```python
from build123d import *

# Parameters (mm, degrees)
BOSS_EXTRUDE1_DEPTH     = 9
SKETCH4_R               = 3.1
BOSS_EXTRUDE3_DEPTH     = 1.75
BOSS_EXTRUDE3_DRAFT     = 35
SKETCH7_R               = 1.600000259
CUT_EXTRUDE4_DEPTH      = 15
CUT_EXTRUDE5_DEPTH      = 7
MIRROR1_START           = -14
MIRROR1_DEPTH           = 4
MIRROR1_START_2         = -18.75
MIRROR1_2_OUTLINE_R     = 1.600000259
MIRROR1_2_DEPTH         = 4.75
CIRPATTERN1_START       = -14
CIRPATTERN1_DEPTH       = 28
CIRPATTERN1_START_2     = -18.75
CIRPATTERN1_2_OUTLINE_R = 1.600000259
CIRPATTERN1_2_DEPTH     = 37.5
CIRPATTERN1_START_3     = -20.405762011
CIRPATTERN1_3_OUTLINE_R = 1.600000259
CIRPATTERN1_3_DEPTH     = 1.655762011
CIRPATTERN1_4_DEPTH     = 28
CIRPATTERN1_5_OUTLINE_R = 1.600000259
CIRPATTERN1_5_DEPTH     = 37.5
CIRPATTERN1_START_4     = 18.75
CIRPATTERN1_6_OUTLINE_R = 1.600000259
CIRPATTERN1_6_DEPTH     = 1.616403084
SKETCH8_R               = 11.1
CUT_EXTRUDE6_DEPTH      = 55.051282913
CUT_EXTRUDE6_TAPER      = 2
SKETCH9_R               = 1.6
CUT_EXTRUDE8_DEPTH      = 55.051282913
CHAMFER1_SIZE           = 1.036815955
CHAMFER1_SIZE_2         = 1


with BuildPart() as part:
    # Sketch3 → Boss-Extrude1 (new body)
    with BuildSketch(Plane.XY):
        with BuildLine():
            Line((-18.75, -34.5), (-18.75, -25.5))
            ThreePointArc((-18.75, -25.5), (-22.155271914, -12.791352203), (-31.458647797, -3.487976321))
            Line((-31.458647797, -3.487976321), (-39.252876431, 1.012023679))
            ThreePointArc((-39.252876431, 1.012023679), (-39.718802257, 1.619230038), (-39.618901834, 2.378049083))
            Line((-39.618901834, 2.378049083), (-36.243901834, 8.223720558))
            ThreePointArc((-36.243901834, 8.223720558), (-35.636695476, 8.689646385), (-34.877876431, 8.589745962))
            Line((-34.877876431, 8.589745962), (-27.9496732, 4.589745962))
            ThreePointArc((-27.9496732, 4.589745962), (-26.811444633, 4.439895328), (-25.900635095, 5.138784068))
            Line((-25.900635095, 5.138784068), (-17.400635095, 19.861215932))
            ThreePointArc((-17.400635095, 19.861215932), (-17.250784461, 20.9994445), (-17.9496732, 21.910254038))
            Line((-17.9496732, 21.910254038), (-24.877876431, 25.910254038))
            ThreePointArc((-24.877876431, 25.910254038), (-25.343802257, 26.517460397), (-25.243901834, 27.276279442))
            Line((-25.243901834, 27.276279442), (-21.868901834, 33.121950917))
            ThreePointArc((-21.868901834, 33.121950917), (-21.261695476, 33.587876743), (-20.502876431, 33.487976321))
            Line((-20.502876431, 33.487976321), (-12.708647797, 28.987976321))
            ThreePointArc((-12.708647797, 28.987976321), (0, 25.582704407), (12.708647797, 28.987976321))
            Line((12.708647797, 28.987976321), (20.502876431, 33.487976321))
            ThreePointArc((20.502876431, 33.487976321), (21.261695476, 33.587876743), (21.868901834, 33.121950917))
            Line((21.868901834, 33.121950917), (25.243901834, 27.276279442))
            ThreePointArc((25.243901834, 27.276279442), (25.343802257, 26.517460397), (24.877876431, 25.910254038))
            Line((24.877876431, 25.910254038), (17.9496732, 21.910254038))
            ThreePointArc((17.9496732, 21.910254038), (17.250784461, 20.9994445), (17.400635095, 19.861215932))
            Line((17.400635095, 19.861215932), (25.900635095, 5.138784068))
            ThreePointArc((25.900635095, 5.138784068), (26.811444633, 4.439895328), (27.9496732, 4.589745962))
            Line((27.9496732, 4.589745962), (34.877876431, 8.589745962))
            ThreePointArc((34.877876431, 8.589745962), (35.636695476, 8.689646385), (36.243901834, 8.223720558))
            Line((36.243901834, 8.223720558), (39.618901834, 2.378049083))
            ThreePointArc((39.618901834, 2.378049083), (39.718802257, 1.619230038), (39.252876431, 1.012023679))
            Line((39.252876431, 1.012023679), (31.458647797, -3.487976321))
            ThreePointArc((31.458647797, -3.487976321), (22.155271914, -12.791352203), (18.75, -25.5))
            Line((18.75, -25.5), (18.75, -34.5))
            ThreePointArc((18.75, -34.5), (18.457106781, -35.207106781), (17.75, -35.5))
            Line((17.75, -35.5), (11, -35.5))
            ThreePointArc((11, -35.5), (10.292893219, -35.207106781), (10, -34.5))
            Line((10, -34.5), (10, -19))
            ThreePointArc((10, -19), (9.560660172, -17.939339828), (8.5, -17.5))
            Line((8.5, -17.5), (-8.5, -17.5))
            ThreePointArc((-8.5, -17.5), (-9.560660172, -17.939339828), (-10, -19))
            Line((-10, -19), (-10, -34.5))
            ThreePointArc((-10, -34.5), (-10.292893219, -35.207106781), (-11, -35.5))
            Line((-11, -35.5), (-17.75, -35.5))
            ThreePointArc((-17.75, -35.5), (-18.457106781, -35.207106781), (-18.75, -34.5))
        make_face()
    extrude(amount=BOSS_EXTRUDE1_DEPTH)


with BuildPart() as boss_extrude3_tool:
    # Sketch4 → Boss-Extrude3 (with draft: the straight prism first)
    with BuildSketch(Plane(origin=(20.5, 0, 0), x_dir=(0, 0, -1), z_dir=(1, 0, 0))):
        with Locations((-4.5, -30)):
            Circle(SKETCH4_R)
    extrude(amount=-BOSS_EXTRUDE3_DEPTH)
    # Boss-Extrude3: the draft: its side faces are tilted about the plane it starts from
    boss_extrude3_sides = [boss_extrude3_tool.faces().sort_by_distance(p)[0] for p in [
        (19.625, -30, 7.6),
    ]]
    draft(boss_extrude3_sides, Plane(origin=(20.5, 0, 0), x_dir=(0, 0, -1), z_dir=(1, 0, 0)), BOSS_EXTRUDE3_DRAFT)


with BuildPart() as part_1:
    add(part.part)

    # Boss-Extrude3: add boss_extrude3_tool
    add(boss_extrude3_tool.part)

    # Sketch7 → Cut-Extrude4 (cut)
    with BuildSketch(Plane(origin=(20.5, 0, 0), x_dir=(0, 0, -1), z_dir=(1, 0, 0))):
        with Locations((-4.5, -30)):
            Circle(SKETCH7_R)
    extrude(amount=-CUT_EXTRUDE4_DEPTH, mode=Mode.SUBTRACT)

    # Sketch5 → Cut-Extrude5 (cut)
    with BuildSketch(Plane(origin=(14, 0, 0), x_dir=(0, 0, -1), z_dir=(1, 0, 0))):
        Polygon((-7.349999794, -28.354551852), (-7.349999794, -31.645448148), (-4.5, -33.290896297), (-1.650000206, -31.645448148), (-1.650000206, -28.354551852), (-4.5, -26.709103703), align=None)
    extrude(amount=-CUT_EXTRUDE5_DEPTH, mode=Mode.SUBTRACT)

    # Mirror1: read off the stored shape, not the designer's step
    # Mirror1 outline → Mirror1 (cut)
    with BuildSketch(Plane.YZ.offset(MIRROR1_START)):
        Polygon((-26.709103703, 4.5), (-28.354551852, 7.349999794), (-31.645448148, 7.349999794), (-33.290896297, 4.5), (-31.645448148, 1.650000206), (-28.354551852, 1.650000206), align=None)
    extrude(amount=MIRROR1_DEPTH, mode=Mode.SUBTRACT)

    # Mirror1 2 outline → Mirror1 2 (cut)
    with BuildSketch(Plane.YZ.offset(MIRROR1_START_2)):
        with Locations((-30, 4.5)):
            Circle(MIRROR1_2_OUTLINE_R)
    extrude(amount=MIRROR1_2_DEPTH, mode=Mode.SUBTRACT)

    # Mirror1 3 outline → Mirror1 3 (revolve)
    with BuildSketch(Plane(origin=(0, -30, 4.5), x_dir=(0, 1, 0), z_dir=(0, 0, -1))):
        Polygon((1.600000259, -18.75), (1.600000259, -20.5), (3.1, -20.5), (4.325363192, -18.75), align=None)
    revolve(axis=Axis((0, -30, 4.5), (1, 0, 0)))

    # CirPattern1: read off the stored shape, not the designer's step
    # CirPattern1 outline → CirPattern1 (cut)
    with BuildSketch(Plane(origin=(0, 0, 0), x_dir=(0.8660254037844362, 0.5000000000000042, 0), z_dir=(0.5000000000000042, -0.8660254037844363, 0)).offset(CIRPATTERN1_START)):
        Polygon((26.709103703, 4.5), (28.354551852, 1.650000206), (31.645448148, 1.650000206), (33.290896297, 4.5), (31.645448148, 7.349999794), (28.354551852, 7.349999794), align=None)
    extrude(amount=CIRPATTERN1_DEPTH, mode=Mode.SUBTRACT)

    # CirPattern1 2 outline → CirPattern1 2 (cut)
    with BuildSketch(Plane(origin=(0, 0, 0), x_dir=(0.8660254037844362, 0.5000000000000042, 0), z_dir=(0.5000000000000042, -0.8660254037844363, 0)).offset(CIRPATTERN1_START_2)):
        with Locations((30, 4.5)):
            Circle(CIRPATTERN1_2_OUTLINE_R)
    extrude(amount=CIRPATTERN1_2_DEPTH, mode=Mode.SUBTRACT)

    # CirPattern1 3 outline → CirPattern1 3 (add)
    with BuildSketch(Plane(origin=(0, 0, 0), x_dir=(0.8660254037844362, 0.5000000000000042, 0), z_dir=(0.5000000000000042, -0.8660254037844363, 0)).offset(CIRPATTERN1_START_3)):
        Polygon((26.709103703, 4.5), (28.354551852, 1.650000206), (31.645448148, 1.650000206), (33.290896297, 4.5), (31.645448148, 7.349999794), (28.354551852, 7.349999794), align=None)
        with Locations((30, 4.5)):
            Circle(CIRPATTERN1_3_OUTLINE_R, mode=Mode.SUBTRACT)
    extrude(amount=CIRPATTERN1_3_DEPTH)

    # CirPattern1 4 outline → CirPattern1 4 (cut)
    with BuildSketch(Plane(origin=(0, 0, 0), x_dir=(0.8660254037844431, -0.4999999999999921, 0), z_dir=(0.4999999999999921, 0.8660254037844433, 0)).offset(CIRPATTERN1_START)):
        Polygon((-26.709103703, -4.5), (-28.354551852, -1.650000206), (-31.645448148, -1.650000206), (-33.290896297, -4.5), (-31.645448148, -7.349999794), (-28.354551852, -7.349999794), align=None)
    extrude(amount=CIRPATTERN1_4_DEPTH, mode=Mode.SUBTRACT)

    # CirPattern1 5 outline → CirPattern1 5 (cut)
    with BuildSketch(Plane(origin=(0, 0, 0), x_dir=(0.8660254037844431, -0.4999999999999921, 0), z_dir=(0.4999999999999921, 0.8660254037844433, 0)).offset(CIRPATTERN1_START_2)):
        with Locations((-30, -4.5)):
            Circle(CIRPATTERN1_5_OUTLINE_R)
    extrude(amount=CIRPATTERN1_5_DEPTH, mode=Mode.SUBTRACT)

    # CirPattern1 6 outline → CirPattern1 6 (add)
    with BuildSketch(Plane(origin=(0, 0, 0), x_dir=(0.8660254037844431, -0.4999999999999921, 0), z_dir=(0.4999999999999921, 0.8660254037844433, 0)).offset(CIRPATTERN1_START_4)):
        Polygon((-26.709103703, -4.5), (-28.354551852, -1.650000206), (-31.645448148, -1.650000206), (-33.290896297, -4.5), (-31.645448148, -7.349999794), (-28.354551852, -7.349999794), align=None)
        with Locations((-30, -4.5)):
            Circle(CIRPATTERN1_6_OUTLINE_R, mode=Mode.SUBTRACT)
    extrude(amount=CIRPATTERN1_6_DEPTH)

    # CirPattern1 7 outline → CirPattern1 7 (revolve)
    with BuildSketch(Plane(origin=(-25.980762114, 15, 4.5), x_dir=(0.8660254037844431, -0.4999999999999921, 0), z_dir=(0, 0, 1))):
        Polygon((3.1, 20.5), (1.600000259, 20.5), (1.600000259, 18.75), (4.325363192, 18.75), align=None)
        Polygon((1.600000259, -18.75), (1.600000259, -20.5), (3.1, -20.5), (4.325363192, -18.75), align=None)
    revolve(axis=Axis((-25.980762114, 15, 4.5), (0.4999999999999921, 0.8660254037844431, 0)))

    # CirPattern1 8 outline → CirPattern1 8 (revolve)
    with BuildSketch(Plane(origin=(25.980762114, 15, 4.5), x_dir=(0.8660254037844362, 0.5000000000000042, 0), z_dir=(0, 0, -1))):
        Polygon((3.1, 20.5), (1.600000259, 20.5), (1.600000259, 18.75), (4.325363192, 18.75), align=None)
        Polygon((1.600000259, -18.75), (1.600000259, -20.5), (3.1, -20.5), (4.325363192, -18.75), align=None)
    revolve(axis=Axis((25.980762114, 15, 4.5), (0.5000000000000042, -0.8660254037844362, 0)))

    # CirPattern1 9 outline → CirPattern1 9 (revolve, cut)
    with BuildSketch(Plane(origin=(-25.980762114, 15, 4.5), x_dir=(0.8660254037844431, -0.4999999999999921, 0), z_dir=(0, 0, 1))):
        Polygon((3.290896297, 20.366403084), (3.193545568, 20.366403084), (3.290896297, 20.227371834), align=None)
    revolve(axis=Axis((-25.980762114, 15, 4.5), (0.4999999999999921, 0.8660254037844431, 0)), mode=Mode.SUBTRACT)

    # CirPattern1 10 outline → CirPattern1 10 (revolve, cut)
    with BuildSketch(Plane(origin=(25.980762114, 15, 4.5), x_dir=(0.8660254037844362, 0.5000000000000042, 0), z_dir=(0, 0, -1))):
        Polygon((3.290896297, -20.227371834), (3.16598615, -20.405762011), (3.290896297, -20.405762011), align=None)
    revolve(axis=Axis((25.980762114, 15, 4.5), (0.5000000000000042, -0.8660254037844362, 0)), mode=Mode.SUBTRACT)

    # Sketch8 → Cut-Extrude6 (cut, through all)
    with BuildSketch(Plane.XY):
        Circle(SKETCH8_R)
    extrude(amount=CUT_EXTRUDE6_DEPTH, taper=CUT_EXTRUDE6_TAPER, mode=Mode.SUBTRACT)

    # Sketch9 → Cut-Extrude8 (cut, through all)
    with BuildSketch(Plane.XY):
        with Locations((13.1, -7.1)):
            Circle(SKETCH9_R)
        with Locations((13.1, 7.1)):
            Circle(SKETCH9_R)
        with Locations((-13.1, 7.1)):
            Circle(SKETCH9_R)
        with Locations((-13.1, -7.1)):
            Circle(SKETCH9_R)
    extrude(amount=CUT_EXTRUDE8_DEPTH, mode=Mode.SUBTRACT)

    # Chamfer1
    # the kernel refuses this chamfer: 1.036815955, 1 mm, written as the material it takes off along each edge
    with BuildSketch(Plane(origin=(0, 0, 0), x_dir=(1, 0, 0), z_dir=(0, 1, 0))) as chamfer1_piece_1:
        Polygon((11.1 + CHAMFER1_SIZE, 0), (11.1 - CHAMFER1_SIZE_2 * 0.0348994967025, -CHAMFER1_SIZE_2 * 0.999390827019), (11.1, 0), align=None)
    revolve(axis=Axis((0, 0, 0), (0, 0, -1)), mode=Mode.SUBTRACT)


solid = part_1.part
```
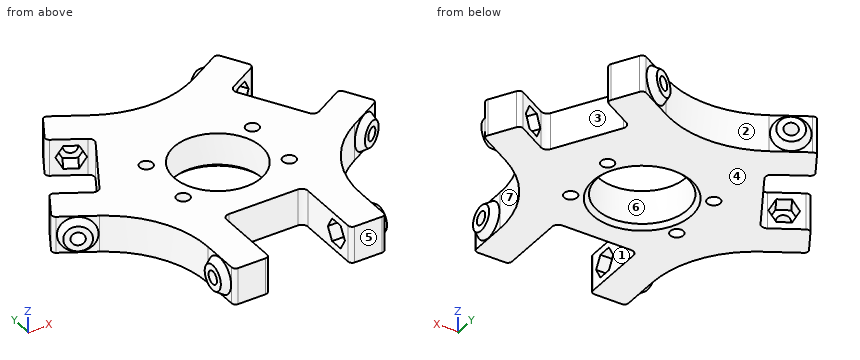
The listing builds one solid part. Answer for the finished solid, in the listing's coordinates (mm). Face numbers are marked on the shaded views. A direction names the side the tool comes from. Coordinates: 2 decimals unless noted, no trailing zeros. Write each loop counter-clockwise with the first axis right and the second up, starting at its lowest first coordinate (ties: lowest second). Pieces come first, ordered by that corner, then holes.
Q1. Given P1, Ø2, axis at x = -25.5, z = 6.5, coming from the +Y side; P2, Ø2.5, axis at y = -28, z = 6, coming from the +X side; P3, Ø3, axis at y = -30.5, z = 4, coming from the -X side, each flat-ended and moving along its own axis, determine where each tip first touches the part or whether it passes through.
Returned:
P1: stops at y = 28.56
P2: stops at x = 20.5
P3: stops at x = -20.5
Q2. The mould has two halves that part along Y. Classify the marked faces 4, 5, 6 and 7: released by +Y, released by -Y, zero draft, split by the parting line, or undercut.
Returned:
face 4: zero draft
face 5: released by -Y
face 6: undercut
face 7: undercut
Q3. Section C-C, the plane y = 13.5 is taken. Write down the section's boundary in (x, z), then the cut area to 3 significant figures.
Returned:
outline: (-21.07, 0) - (21.07, 0) - (21.07, 9) - (-21.07, 9) - close
area: 379 mm2
Q4. Find the intervals of material crossed by line 1 along X through (y, z) = (0, 5.25); line 2 along X through (y, z) = (7.1, 2.75); line 3 along X through (y, z) = (-7.1, 6.75), in increasing order.
Returned:
line 1: x = -38.96 to -36.27, -33.01 to -10.92, 10.92 to 33.01, 36.27 to 38.96
line 2: x = -36.89 to -33.18, -24.77 to -14.7, -11.5 to -8.41, 8.41 to 11.5, 14.7 to 24.77, 33.18 to 36.89
line 3: x = -26.63 to -14.7, -11.5 to -8.22, 8.22 to 11.5, 14.7 to 26.63
Q5. Section A-A, the plane x = 0 is taken. Write down the section's boundary in (y, z), then the cut area to 3 significant figures.
Returned:
outline: (-17.5, 0) - (-12.14, 0) - (-11.07, 1) - (-10.79, 9) - (-17.5, 9) - close; (10.79, 9) - (11.07, 1) - (12.14, 0) - (25.58, 0) - (25.58, 9) - close
area: 190 mm2
Q6. Section B-B, the plane y = -7.1 is taken. Give the number of separate pieces and of enclosed holes in the cut face, then the cut area to 3 significant figures.
Returned:
separate pieces: 4
enclosed holes: 0
area: 271 mm2
Q7. Section D-D, the plane y = 21 is taken. Write down the section's boundary in (x, z).
Returned:
outline: (-17.25, 0) - (17.25, 0) - (17.25, 9) - (-17.25, 9) - close
Q8. Which of the six approach directions +Z, -Z, +X, -X, +Y, -Y give full straight-line access (tool end or side, diameter ignored) to the marked faces 1, 2 and 3?
Returned:
face 1: +Z, -Z, -Y
face 2: +Z, -Z, +Y
face 3: +Z, -Z
